Design review of the part built by this model. Coordinates are the model's own, in mm. A direction names the side the tool comes from. Coordinates: 2 decimals unless noted, no trailing zeros. Order: outer loops, then holes, each group sorted by start corner. A loop starts at its lowest first (then second) coordinate and runs counter-clockwise, first axis right, second up. Notation, with made-up numbers: (-27, 14) -> (2, 14) arc R16 ccw to (2, 33) -> close; hole circle Ø2 at (27, 57). An arc over 180 degrees is marked (long way). Write item = value, one per line.
```python
from build123d import *

# Parameters (mm, degrees)
BOSS_EXTRUDE1_DEPTH            = 130
FILLET1_R                      = 4
FILLET2_R                      = 7
SKETCH2_R                      = 8.5
CUT_EXTRUDE1_DEPTH             = 100
M3_CLEARANCE_HOLE1_D           = 3.2
M3_CLEARANCE_HOLE1_CSINK_D     = 3.25
M3_CLEARANCE_HOLE1_CSINK_ANGLE = 90
M4_CLEARANCE_HOLE1_D           = 4.3
M4_CLEARANCE_HOLE1_DEPTH       = 100
M4_CLEARANCE_HOLE1_TIP         = 1.291850331
M5_CLEARANCE_HOLE2_D           = 5.3
M5_CLEARANCE_HOLE2_DEPTH       = 100
M5_CLEARANCE_HOLE2_TIP         = 1.59228064


with BuildPart() as part:
    # Sketch1 → Boss-Extrude1 (new body)
    with BuildSketch(Plane.XY):
        Polygon((0, 4), (26, 4), (26, 106), (156, 106), (156, 4), (182, 4), (182, 0), (152, 0), (152, 102), (30, 102), (30, 0), (0, 0), align=None)
    extrude(amount=BOSS_EXTRUDE1_DEPTH)

    # Fillet1
    fillet1_edges = [part.edges().sort_by_distance(p)[0] for p in [
        (26, 4, 65),
        (156, 4, 65),
        (152, 102, 65),
        (30, 102, 65),
    ]]
    fillet(fillet1_edges, radius=FILLET1_R)

    # Fillet2
    fillet2_edges = [part.edges().sort_by_distance(p)[0] for p in [
        (26, 106, 65),
        (156, 106, 65),
        (152, 0, 65),
        (30, 0, 65),
    ]]
    fillet(fillet2_edges, radius=FILLET2_R)

    # Sketch2 → Cut-Extrude1 (cut)
    with BuildSketch(Plane(origin=(0, 106, 0), x_dir=(1, 0, 0), z_dir=(0, 1, 0))):
        with Locations((91, -65)):
            Circle(SKETCH2_R)
    extrude(amount=-CUT_EXTRUDE1_DEPTH, mode=Mode.SUBTRACT)

    # M3 Clearance Hole1 (through all)
    with Locations(Plane(origin=(0, 106, 0), x_dir=(1, 0, 0), z_dir=(0, 1, 0))):
        with Locations((91, -54), (100.526279442, -59.5), (100.526279442, -70.5), (91, -76), (81.473720558, -70.5), (81.473720558, -59.5), (91, -65)):
            CounterSinkHole(M3_CLEARANCE_HOLE1_D / 2, M3_CLEARANCE_HOLE1_CSINK_D / 2, counter_sink_angle=M3_CLEARANCE_HOLE1_CSINK_ANGLE)

    # M4 Clearance Hole1
    with Locations(Plane(origin=(0, 106, 0), x_dir=(1, 0, 0), z_dir=(0, 1, 0))):
        with Locations((137, -65), (114, -104.837168574), (68, -104.837168574), (45, -65), (68, -25.162831426), (114, -25.162831426), (91, -65)):
            Hole(M4_CLEARANCE_HOLE1_D / 2, depth=M4_CLEARANCE_HOLE1_DEPTH)
            with Locations((0, 0, -(M4_CLEARANCE_HOLE1_DEPTH + M4_CLEARANCE_HOLE1_TIP / 2))):  # 118° drill point
                Cone(0, M4_CLEARANCE_HOLE1_D / 2, M4_CLEARANCE_HOLE1_TIP, mode=Mode.SUBTRACT)

    # M5 Clearance Hole2
    with Locations(Plane(origin=(0, 4, 0), x_dir=(1, 0, 0), z_dir=(0, 1, 0))):
        with Locations((11, -15), (11, -115), (171, -115), (171, -15)):
            Hole(M5_CLEARANCE_HOLE2_D / 2, depth=M5_CLEARANCE_HOLE2_DEPTH)
            with Locations((0, 0, -(M5_CLEARANCE_HOLE2_DEPTH + M5_CLEARANCE_HOLE2_TIP / 2))):  # 118° drill point
                Cone(0, M5_CLEARANCE_HOLE2_D / 2, M5_CLEARANCE_HOLE2_TIP, mode=Mode.SUBTRACT)


solid = part.part
```
(1) We need section B-B (x = 45). Write out the cut boundary in (y, z), and give its area (3 significant figures).
Report:
outline = (102, 0) -> (106, 0) -> (106, 62.85) -> (102, 62.85) -> close; (102, 67.15) -> (106, 67.15) -> (106, 130) -> (102, 130) -> close
area = 503 mm²
(2) For faces 1 (the cylindrical face through (154, 2.1, 65.9)), 2 (the flat face through (11, 4, 64)), 3 (the cylindrical face through (111.95, 103.97, 104.19)), list the 3-axis set-ups (+Z, -Z, +X, -X, +Y, -Y) from which the entire face can be reached by the end or side of a thin tool; tool diameter is ignored.
Report:
face_1 = +Z, -Z, -Y
face_2 = +Z, -Z, -X, +Y
face_3 = +Y, -Y
(3) We need section C-C (y = 19). Write out the cut boundary in (x, z), and give its area (3 significant figures).
Report:
outline = (26, 0) -> (30, 0) -> (30, 130) -> (26, 130) -> close; (152, 0) -> (156, 0) -> (156, 130) -> (152, 130) -> close
area = 1,040 mm²
(4) We need section D-D (z = 115). Write out the cut boundary in (x, y).
Report:
outline = (0, 0) -> (8.35, 0) -> (8.35, 4) -> (0, 4) -> close; (13.65, 0) -> (23, 0) arc R7 ccw to (30, 7) -> (30, 98) arc R4 cw to (34, 102) -> (148, 102) arc R4 cw to (152, 98) -> (152, 7) arc R7 ccw to (159, 0) -> (168.35, 0) -> (168.35, 4) -> (160, 4) arc R4 cw to (156, 8) -> (156, 99) arc R7 ccw to (149, 106) -> (33, 106) arc R7 ccw to (26, 99) -> (26, 8) arc R4 cw to (22, 4) -> (13.65, 4) -> close; (173.65, 0) -> (182, 0) -> (182, 4) -> (173.65, 4) -> close
(5) We need section A-A (z = 65). Give the number of separate pieces and of enclosed holes in the cut face, and give its area (3 significant figures).
Report:
separate_pieces = 4
enclosed_holes = 0
area = 1,410 mm²
(6) Insertion check: pin 1 (5 mm diameter, centred on x = 108, z = 68.5, fed in from -Y); pin 2 (1.5 mm diameter, centred on y = 81.5, z = 16.5, fed in from +X); pin 3 (6 mm diameter, centred on x = 171, z = 115, fed in from +Y). Each pin has a flat end and moves straight along its axis. Give the tip position at first contact, or say it passes through.
Report:
pin_1 = 102
pin_2 = 156
pin_3 = 4
(7) The part is to be moulded in two halves that separate along X. For faces 4 (the flat face through (103, 106, 64)), 5 (the flat face through (156, 54, 64)), 6 (the cylindrical face through (11.34, 1.97, 112.37)), 7 (the flat face through (26, 53, 64)), say which applies: released by +X, released by -X, zero draft, split by the parting line, or undercut.
Report:
face_4 = zero draft
face_5 = released by +X
face_6 = undercut
face_7 = released by -X
(8) For L1, parallel to Z at x = 91, y = 103.3; L2, parallel to X at y = 94, z = 18.5; L3, parallel to X at y = 104.85, z = 59.5, list the stretches that pass through material, from the lowest coordinate up.
Report:
L1 = 0 to 52.4, 55.6 to 56.5, 73.5 to 74.4, 77.6 to 130
L2 = 26 to 30, 152 to 156
L3 = 29.16 to 79.87, 83.07 to 84.52, 97.48 to 98.93, 102.13 to 152.84
